```python
from build123d import *

# Parameters (mm, degrees)
F4_DEPTH = 23.8


with BuildPart() as f2:
    # F2: sweep along a path in F1
    with BuildLine(Plane.XY) as f2_path:
        Line((100, 0), (92.191627, 23.749301))
    # F0 (on Front) → F2 (sweep)
    with BuildSketch(Plane.XZ):
        Polygon((100, 29), (0, 29), (0, 26), (97, 26), (97, 3), (0, 3), (0, 0), (100, 0), align=None)
    sweep(path=f2_path.line)

    # F3 (on Front) → F4 (join)
    with BuildSketch(Plane.XZ):
        Polygon((68.705302, -11.464806), (68.705302, 0), (65.705302, 0), (65.705302, -11.963572), (66.974133, -13.332377), align=None)
        Polygon((68.705302, -73.235512), (68.705302, -11.464806), (66.974133, -13.332377), (65.705302, -11.963572), (65.705302, -80), (109.149036, -80), (115.005407, -64.447597), (111.799763, -64.447597), (108.102038, -74.267415), (107.073064, -77), (104.542602, -77), (72.230041, -77), (68.705302, -77), align=None)
        Polygon((79.33275, 0), (68.705302, 0), (68.705302, -11.464806), align=None)
        Polygon((65.705302, -11.963572), (65.705302, 0), (54.615512, 0), align=None)
        Polygon((72.230041, -77), (68.705302, -73.235512), (68.705302, -77), align=None)
        Polygon((108.102038, -74.267415), (104.542602, -77), (107.073064, -77), align=None)
    extrude(amount=-F4_DEPTH)


solid = f2.part
```
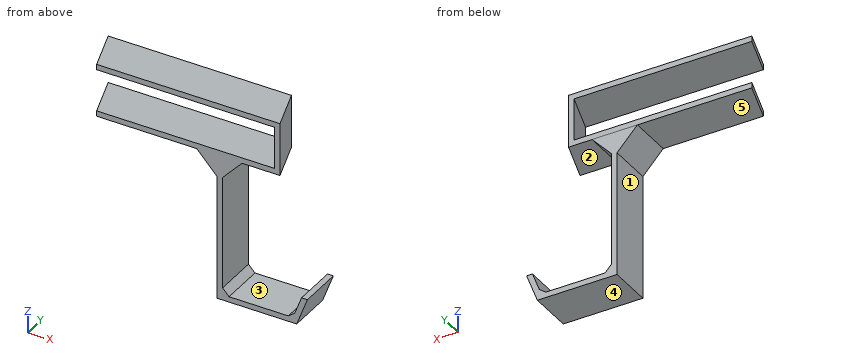
Verification items for the finished model (mm, model axes). Face numbers are marked on the shaded views. A direction names the side the tool comes from. Coordinates: 2 decimals unless noted, no trailing zeros. Loops run counter-clockwise (first coordinate to the right, second up) from the corner with the lowest first, then second, coordinate; pieces in that order, holes last. Notation, with made-up numbers: (79.25, 16.5) - (95.25, 16.5) arc R25 cw to (95.25, 30.5) - close; hole circle Ø7 at (35, 47). An arc over 180 degrees is marked (long way). Put each result on its own line as item: value.
Item 1: Section check A-A (x = 81.5). Enter the section's corners in (y, z).
Conclusion:
outline: (0, -80) - (23.8, -80) - (23.8, -77) - (0, -77) - close; (0, 0) - (23.75, 0) - (23.75, 3) - (0, 3) - close; (0, 26) - (23.75, 26) - (23.75, 29) - (0, 29) - close
Item 2: Section check D-D (y = 19.5). Enter the section's corners in (x, z), then the cut area to 3 significant figures.
Conclusion:
outline: (-6.41, 0) - (54.62, 0) - (65.71, -11.96) - (65.71, -80) - (109.15, -80) - (115.01, -64.45) - (111.8, -64.45) - (108.1, -74.27) - (104.54, -77) - (72.23, -77) - (68.71, -73.24) - (68.71, -11.46) - (79.33, 0) - (93.59, 0) - (93.59, 29) - (-6.41, 29) - (-6.41, 26) - (90.59, 26) - (90.59, 3) - (-6.41, 3) - close
area: 1,210 mm2
Item 3: Scan lines: line 1 along Z through (x, y) = (81, 12); line 2 along X through (y, z) = (14.5, -64.5); line 3 along Z through (x, y) = (19, 11.75). Record each from-to range of solid material in increasing order.
Conclusion:
line 1: z = -80 to -77, 0 to 3, 26 to 29
line 2: x = 65.71 to 68.71, 111.78 to 114.99
line 3: z = 0 to 3, 26 to 29
Item 4: Section check B-B (x = 35.5). Enter the section's corners in (y, z), then the cut area to 3 significant figures.
Conclusion:
outline: (0, 0) - (23.75, 0) - (23.75, 3) - (0, 3) - close; (0, 26) - (23.75, 26) - (23.75, 29) - (0, 29) - close
area: 142 mm2
Item 5: Gauge pin test, flat ends, axial feed: pin 1 Ø12 at (y, z) = (13, -37.5) entering from +X; pin 2 Ø14.5 at (x, z) = (53.5, 10) entering from +Y; pin 3 Ø6 at (x, y) = (57.5, 2.5) entering from -Z. Record the tip position at first contact, or that the pin passes through.
Conclusion:
pin 1: stops at x = 68.71
pin 2: stops at y = 23.75
pin 3: stops at z = -6.35
Item 6: Section check C-C (z = -70.5). Enter the section's corners in (x, y).
Conclusion:
outline: (65.71, 0) - (68.71, 0) - (68.71, 23.8) - (65.71, 23.8) - close; (109.52, 0) - (112.73, 0) - (112.73, 23.8) - (109.52, 23.8) - close
Item 7: Draft check along X on the marked faces 1, 2 and 3. Enter one of: pulls with the +X half, pulls with the -X half, needs draft (parallel to the pull), parting line crosses it, or undercut.
Conclusion:
face 1: pulls with the -X half
face 2: needs draft
face 3: undercut
Item 8: Set-up check for the marked faces 4 and 5: record each of +Z, -Z, +X, -X, +Y, -Y from which the full face is reachable in a straight line by a thin tool's end or side.
Conclusion:
face 4: -Z, +X, -X, +Y, -Y
face 5: -Z, -X, +Y, -Y
